```python
from build123d import *

# Parameters (mm, degrees)
BOSS_EXTRUDE1_DEPTH = 3
CUT_EXTRUDE1_REACH  = 5
SKETCH2_R           = 5


with BuildPart() as part:
    # Sketch1 → Boss-Extrude1 (new body)
    with BuildSketch(Plane.XY):
        Polygon((-26.901408451, -70.281690141), (53.098591549, 129.718309859), (-106.901408451, 129.718309859), align=None)
    extrude(amount=BOSS_EXTRUDE1_DEPTH)

    # Sketch2 → Cut-Extrude1 (cut, up to next)
    with BuildSketch(Plane.XY.offset(3), mode=Mode.PRIVATE) as cut_extrude1_sk1:
        with Locations((-26.901408451, 94.718309859)):
            Circle(SKETCH2_R)
    cut_extrude1_tool1 = extrude(cut_extrude1_sk1.sketch, amount=-CUT_EXTRUDE1_REACH, mode=Mode.PRIVATE) & part.part
    add(cut_extrude1_tool1.solids().sort_by_distance((-26.901408, 94.71831, 3))[0], mode=Mode.SUBTRACT)
    # Sketch2 → Cut-Extrude1 (cut, up to next)
    with BuildSketch(Plane.XY.offset(3), mode=Mode.PRIVATE) as cut_extrude1_sk2:
        with Locations((-26.901408451, 69.718309859)):
            Circle(SKETCH2_R)
    cut_extrude1_tool2 = extrude(cut_extrude1_sk2.sketch, amount=-CUT_EXTRUDE1_REACH, mode=Mode.PRIVATE) & part.part
    add(cut_extrude1_tool2.solids().sort_by_distance((-26.901408, 69.71831, 3))[0], mode=Mode.SUBTRACT)


solid = part.part
```
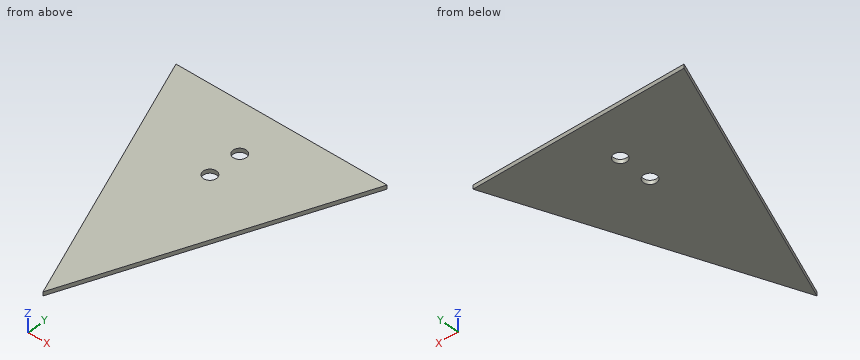
Check sheet for the modelled part. Datum: model origin and axes. Units: mm. Coordinates: 2 decimals unless noted, no trailing zeros. Order: outer loops, then holes, each group sorted by start corner. A loop starts at its lowest first (then second) coordinate and runs counter-clockwise, first axis right, second up. Notation, with made-up numbers: M 72,-24 L 127,-24 A36 ccw 127,14 Z; hole C -27.75,51.25 d1. An arc over 180 degrees is marked long. Write each question's results on one line, items separated by ' | '. Start each with the question number.
1. Cross-section at B-B on y = 37. Record the cut outline in (x, z).
2. Cross-section at C-C on x = -41.5. Record the cut outline in (y, z).
3. Cross-section at A-A on z = 2.55. Record the cut outline in (x, y).
4. Material ranges on probe 1 along X at (y, z) = (73, 0.5); probe 2 along X at (y, z) = (109, 1.25); probe 3 along X at (y, z) = (59.5, 1.05), recorded low to high.
5. Go/stop test with a flat-tipped pin: P1, Ø8, axis at x = -26.9, y = 69.72, coming from the +Z side. Record where the tip stops, or that it passes through.
Checks:
1) outline: M -69.81,0 L 16.01,0 L 16.01,3 L -69.81,3 Z
2) outline: M -33.79,0 L 129.72,0 L 129.72,3 L -33.79,3 Z
3) outline: M -106.9,129.72 L -26.9,-70.28 L 53.1,129.72 Z; hole C -26.9,69.72 d10; hole C -26.9,94.72 d10
4) probe 1: x = -84.21 to -30.67, -23.13 to 30.41 | probe 2: x = -98.61 to 44.81 | probe 3: x = -78.81 to 25.01
5) P1: passes through
